```python
from build123d import *

# Parameters (mm, degrees)
SKETCH1_W           = 39
SKETCH1_H           = 13
BOSS_EXTRUDE1_DEPTH = 3
SKETCH5_W           = 39
SKETCH5_H           = 9
CUT_EXTRUDE1_DEPTH  = 2
SKETCH2_W           = 1
SKETCH2_H           = 9
BOSS_EXTRUDE2_DEPTH = 1
SKETCH6_R           = 1.65
CUT_EXTRUDE2_DEPTH  = 4


with BuildPart() as part:
    # Sketch1 → Boss-Extrude1 (new body)
    with BuildSketch(Plane(origin=(0, 0, 0), x_dir=(1, 0, 0), z_dir=(0, 1, 0))):
        Rectangle(SKETCH1_W, SKETCH1_H)
    extrude(amount=BOSS_EXTRUDE1_DEPTH)

    # Sketch5 → Cut-Extrude1 (cut)
    with BuildSketch(Plane(origin=(0, 3, 0), x_dir=(1, 0, 0), z_dir=(0, 1, 0))):
        Rectangle(SKETCH5_W, SKETCH5_H)
    extrude(amount=-CUT_EXTRUDE1_DEPTH, mode=Mode.SUBTRACT)

    # Sketch2 → Boss-Extrude2 (add)
    with BuildSketch(Plane(origin=(0, 1, 0), x_dir=(1, 0, 0), z_dir=(0, 1, 0))):
        with Locations((7, 0)):
            Rectangle(SKETCH2_W, SKETCH2_H)
        with Locations((5, 0)):
            Rectangle(SKETCH2_W, SKETCH2_H)
        with Locations((9, 0)):
            Rectangle(SKETCH2_W, SKETCH2_H)
        with Locations((3, 0)):
            Rectangle(SKETCH2_W, SKETCH2_H)
        with Locations((11, 0)):
            Rectangle(SKETCH2_W, SKETCH2_H)
        with Locations((13, 0)):
            Rectangle(SKETCH2_W, SKETCH2_H)
        with Locations((15, 0)):
            Rectangle(SKETCH2_W, SKETCH2_H)
        with Locations((-3, 0)):
            Rectangle(SKETCH2_W, SKETCH2_H)
        with Locations((17, 0)):
            Rectangle(SKETCH2_W, SKETCH2_H)
        with Locations((-5, 0)):
            Rectangle(SKETCH2_W, SKETCH2_H)
        with Locations((19, 0)):
            Rectangle(SKETCH2_W, SKETCH2_H)
        with Locations((-7, 0)):
            Rectangle(SKETCH2_W, SKETCH2_H)
        with Locations((-9, 0)):
            Rectangle(SKETCH2_W, SKETCH2_H)
        with Locations((-11, 0)):
            Rectangle(SKETCH2_W, SKETCH2_H)
        with Locations((-13, 0)):
            Rectangle(SKETCH2_W, SKETCH2_H)
        with Locations((-15, 0)):
            Rectangle(SKETCH2_W, SKETCH2_H)
        with Locations((-17, 0)):
            Rectangle(SKETCH2_W, SKETCH2_H)
        with Locations((-19, 0)):
            Rectangle(SKETCH2_W, SKETCH2_H)
    extrude(amount=BOSS_EXTRUDE2_DEPTH)

    # Sketch6 → Cut-Extrude2 (cut, through all)
    with BuildSketch(Plane.XZ):
        Circle(SKETCH6_R)
    extrude(amount=-CUT_EXTRUDE2_DEPTH, mode=Mode.SUBTRACT)


solid = part.part
```
The listing builds one solid part. Answer for the finished solid, in the listing's coordinates (mm). A direction names the side the tool comes from. Give positions to 0.01 mm unless a question says otherwise; leave off trailing zeros. Order: outer loops, then holes, each group sorted by start corner. A loop starts at its lowest first (then second) coordinate and runs counter-clockwise, first axis right, second up.
Item 1: Which of the six approach directions +Z, -Z, +X, -X, +Y, -Y give full straight-line access (tool end or side, diameter ignored) to faces 5 (the face through (-7, 2, 0)), 6 (the face through (-7.5, 1.5, 0.1)), 7 (the face through (0, 3, -6))?
From the geometry:
face 5: +X, -X, +Y
face 6: +Y
face 7: +Z, -Z, +X, -X, +Y
Item 2: The part is cut by section C-C, the plane x = 8. Give the vertices of the cut face in (y, z).
From the geometry:
outline: (0, -6.5) - (3, -6.5) - (3, -4.5) - (1, -4.5) - (1, 4.5) - (3, 4.5) - (3, 6.5) - (0, 6.5) - close
Item 3: Find the intervals of material crossed by probe 1 along Z at (x, y) = (-4, 2.05); probe 2 along Z at (x, y) = (0, 0.55); probe 3 along Y at (x, z) = (11, -1.5), in increasing order.
From the geometry:
probe 1: z = -6.5 to -4.5, 4.5 to 6.5
probe 2: z = -6.5 to -1.65, 1.65 to 6.5
probe 3: y = 0 to 2
Item 4: The part is cut by section B-B, the plane y = 0.4. Give the vertices of the cut face in (x, z).
From the geometry:
outline: (-19.5, -6.5) - (19.5, -6.5) - (19.5, 6.5) - (-19.5, 6.5) - close; hole circle Ø3.3 at (0, 0)
Item 5: For a pull along X with two mould halves and no side action, classify faces 1 (the face through (6, 1, 0)), 2 (the face through (17, 2, 0)), 3 (the face through (19.5, 1, 0)), 4 (the face through (2.5, 1.5, 0.1)) as pulls with the +X half, pulls with the -X half, needs draft (parallel to the pull), parting line crosses it, or undercut.
From the geometry:
face 1: undercut
face 2: needs draft
face 3: pulls with the +X half
face 4: undercut
Item 6: The part is cut by section A-A, the plane x = 0. Give the vertices of the cut face in (y, z), and give its area (3 significant figures).
From the geometry:
outline: (0, -6.5) - (3, -6.5) - (3, -4.5) - (1, -4.5) - (1, -1.65) - (0, -1.65) - close; (0, 1.65) - (1, 1.65) - (1, 4.5) - (3, 4.5) - (3, 6.5) - (0, 6.5) - close
area: 17.7 mm2
Item 7: Given pin 1 Ø0.5 at (x, z) = (7, 0) entering from +Y; pin 2 Ø2.5 at (x, z) = (0, 0) entering from -Y; pin 3 Ø0.5 at (x, z) = (14, 2) entering from +Y, each flat-ended and moving along its own axis, determine where each tip first touches the part or whether it passes through.
From the geometry:
pin 1: stops at y = 2
pin 2: passes through
pin 3: stops at y = 1
